Solid Edge part; units mm, degrees
sketch "Sketch1" plane through (0, 0, 0) normal (0, -1, 0) x (1, 0, 0)
  line L0 (0, 10) -> (27.5, 10)
  line L1 (27.5, 10) -> (27.5, 0)
  line L2 (27.5, 0) -> (0, 0)
  dimension "D1" = 27.5
revolve "RevolvedProtrusion1" add sketch "Sketch1" angle 360 about axis through (0, 0, 0) along (0, 0, 1)
chamfer "Chamfer1" distance 2.5 angle 45 1 edges at (-27.5, 0, 0)
hole "Hole_1" at (-13, 13, 0) direction (0, 0, 1) diameter 5 end up to next
hole "Hole1" at (-13, -13, 0) direction (0, 0, 1) diameter 5 end up to next
hole "Hole2" at (13, 13, 0) direction (0, 0, 1) diameter 5 end up to next
hole "Hole3" at (13, -13, 0) direction (0, 0, 1) diameter 5 end up to next
hole "Hole_5" at (0, 0, 0) direction (0, 0, 1) diameter 5.6 depth 6 tip angle 118
chamfer "Chamfer_2" distance 0.5 angle 45 1 edges at (0, -2.8, 0)
sketch "Sketch2" plane through (0, 0, 0) normal (0, 0, -1) x (-1, 0, 0)
  line L0 (-16.5, 15.0207) -> (-16.5, 10.9793)
  line L1 (-16.5, 10.9793) -> (-13, 8.9585)
  line L2 (-13, 8.9585) -> (-9.5, 10.9793)
  line L3 (-9.5, 10.9793) -> (-9.5, 15.0207)
  line L4 (-9.5, 15.0207) -> (-13, 17.0415)
  line L5 (-13, 17.0415) -> (-16.5, 15.0207)
extrude "ExtrudedCutout_1" cut sketch "Sketch2" against normal blind 5
chamfer "Chamfer_3" distance 0.5 angle 45 6 edges at (14.75, 16.0311, 0) (11.25, 16.0311, 0) (9.5, 13, 0) (11.25, 9.9689, 0) (14.75, 9.9689, 0) (16.5, 13, 0)
mirror "Mirror1" about plane through (0, 0, 0) normal (1, 0, 0) of "ExtrudedCutout_1"
chamfer "Chamfer2" distance 0.5 angle 45 6 edges at (-14.75, 16.0311, 0) (-11.25, 16.0311, 0) (-9.5, 13, 0) (-11.25, 9.9689, 0) (-14.75, 9.9689, 0) (-16.5, 13, 0)
mirror "Mirror2" about plane through (0, 0, 0) normal (0, -1, 0) of "ExtrudedCutout_1", "Mirror1"
chamfer "Chamfer3" distance 0.5 angle 45 6 edges at (14.75, -16.0311, 0) (11.25, -16.0311, 0) (9.5, -13, 0) (11.25, -9.9689, 0) (14.75, -9.9689, 0) (16.5, -13, 0)
chamfer "Chamfer4" distance 0.5 angle 45 6 edges at (-14.75, -16.0311, 0) (-11.25, -16.0311, 0) (-9.5, -13, 0) (-11.25, -9.9689, 0) (-14.75, -9.9689, 0) (-16.5, -13, 0)
properties material "Polyethylene, low density"
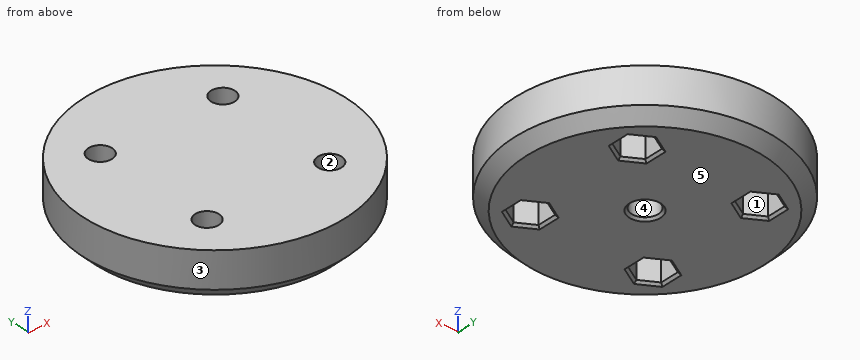
Verification items for the finished model (mm, model axes). Face numbers are marked on the shaded views. A direction names the side the tool comes from. Give positions to 0.01 mm unless a question says otherwise; leave off trailing zeros. Loops run counter-clockwise (first coordinate to the right, second up) from the corner with the lowest first, then second, coordinate; pieces in that order, holes last.
1. Go/stop test with flat-tipped pins: pin 1 Ø3.5 at (x, y) = (-12.5, -11) entering from -Z; pin 2 Ø4.5 at (y, z) = (13, 2) entering from -X; pin 3 Ø2 at (y, z) = (-13, 2) entering from +X; pin 4 Ø4.5 at (x, y) = (-13, -13) entering from -Z. Record where each tip stops, or that it passes through.
2. Section check B-B, the plane z = 8.5. Enter the section's corners in (x, y), then the cut area to 3 significant figures.
3. Section check A-A, the plane z = 4. Enter the section's corners in (x, y).
4. Mould release check, pull along Y, two halves, no side actions. Record for the marked faces 3, 4 and 5: released by +Y, released by -Y, zero draft, split by the parting line, or undercut.
5. Set-up check for the marked faces 1 and 2: record each of +Z, -Z, +X, -X, +Y, -Y from which the full face is reachable in a straight line by a thin tool's end or side.
6. Thickness scan on line 1 (X direction, y = -13.5, z = 2.5); line 2 (Y direction, x = -15.5, z = 3); line 3 (X direction, y = -13, z = 8.1). Record the ranges inside material, lowest first.
7. Section check C-C, the plane y = -13. Count the separate pieces of the cut face and the enclosed holes in it, then the cut area to 3 significant figures.
Geometry says:
1. pin 1: stops at z = 0.27
1. pin 2: stops at x = -25.29
1. pin 3: stops at x = 24.68
1. pin 4: passes through
2. outline: circle Ø55 at (0, 0); hole circle Ø5 at (-13, -13); hole circle Ø5 at (-13, 13); hole circle Ø5 at (13, -13); hole circle Ø5 at (13, 13)
2. area: 2,300 mm2
3. outline: circle Ø55 at (0, 0); hole (-16.5, -15.02) - (-13, -17.04) - (-9.5, -15.02) - (-9.5, -10.98) - (-13, -8.96) - (-16.5, -10.98) - close; hole (-16.5, 10.98) - (-13, 8.96) - (-9.5, 10.98) - (-9.5, 15.02) - (-13, 17.04) - (-16.5, 15.02) - close; hole circle Ø5.6 at (0, 0); hole (9.5, -15.02) - (13, -17.04) - (16.5, -15.02) - (16.5, -10.98) - (13, -8.96) - (9.5, -10.98) - close; hole (9.5, 10.98) - (13, 8.96) - (16.5, 10.98) - (16.5, 15.02) - (13, 17.04) - (9.5, 15.02) - close
4. face 3: split by the parting line
4. face 4: undercut
4. face 5: zero draft
5. face 1: -Z
5. face 2: +Z, -Z
6. line 1: x = -23.96 to -16.5, -9.5 to 9.5, 16.5 to 23.96
6. line 2: y = -22.72 to -15.6, -10.4 to 10.4, 15.6 to 22.72
6. line 3: x = -24.23 to -15.5, -10.5 to 10.5, 15.5 to 24.23
7. separate pieces: 3
7. enclosed holes: 0
7. area: 357 mm2
